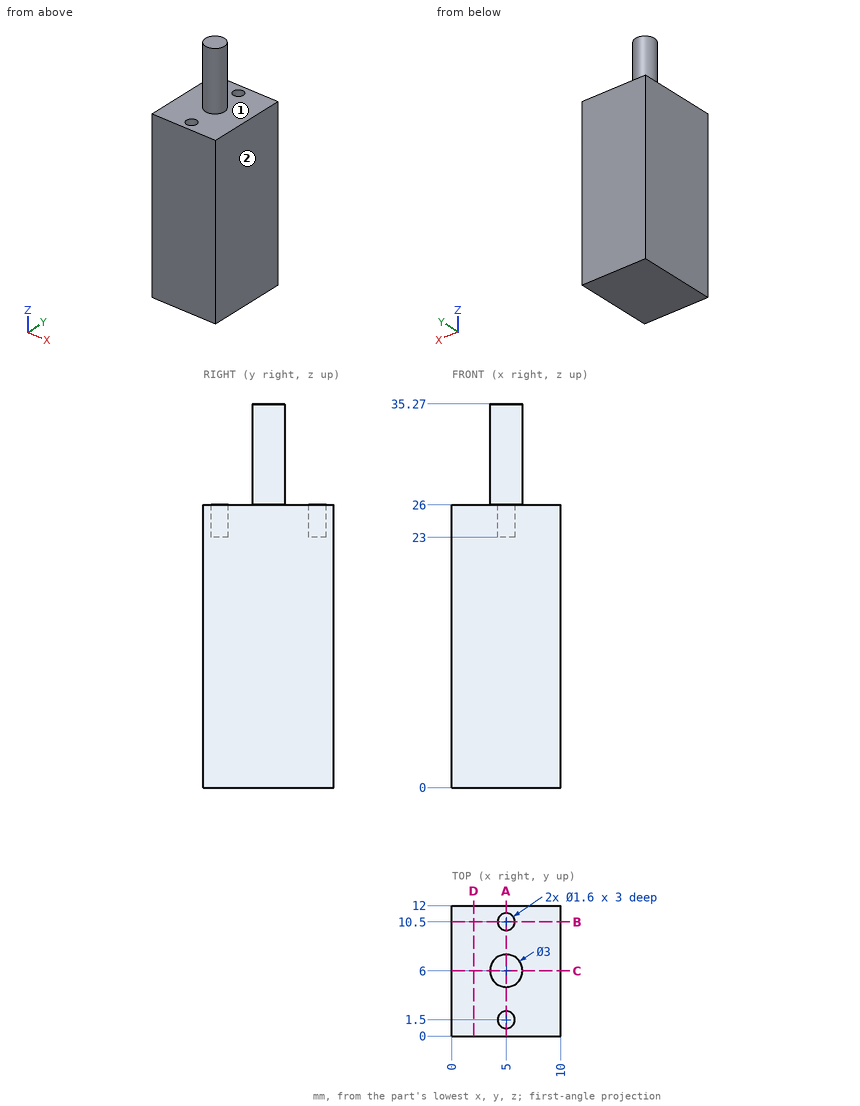
Here's the drawing with two shaded views (mm, measured from the low corner). I have some questions. A direction names the side the tool comes from. Coordinates: 2 decimals unless noted, no trailing zeros. Write each loop counter-clockwise with the first axis right and the second up, starting at its lowest first coordinate (ties: lowest second). Pieces come first, ordered by that corner, then holes. Notation, with made-up numbers: (4, -5) -> (49, -5) arc R34 ccw to (49, 34) -> close; hole circle Ø9 at (46.5, 20.5). An arc over 180 degrees is marked (long way). One line per question, with ' | ' between items. Start each with the question number.
1. If we section it at D-D (x = 2): Please give me the cut outline in (y, z).
2. Please list where these lines run through material, in increasing order: line 1 along Y through (x, z) = (5, 24.15); line 2 along Z through (x, y) = (6.25, 5); line 3 along X through (y, z) = (6.75, 26.5).
3. Will these pins go through, and if not, where does the flat tip stop? P1, Ø1.8, axis at x = 5, y = 10.5, coming from the +Z side; P2, Ø4, axis at y = 8, z = 31, coming from the -X side; P3, Ø3, axis at x = 3.5, y = 7.5, coming from the +Z side.
4. For the marked faces 1 and 2, which set-ups out of +Z, -Z, +X, -X, +Y, -Y let a thin tool reach every point of the face, with its end or its side?
5. If we section it at B-B (y = 10.5): Please give me the cut outline in (x, z), and give its area (3 significant figures).
6. If we section it at C-C (y = 6): Please give me the cut outline in (x, z).
7. If we section it at A-A (x = 5): Please give me the cut outline in (y, z).
Return value:
1) outline: (0, 0) -> (12, 0) -> (12, 26) -> (0, 26) -> close
2) line 1: y = 0 to 0.7, 2.3 to 9.7, 11.3 to 12 | line 2: z = 0 to 26 | line 3: x = 3.7 to 6.3
3) P1: stops at z = 26 | P2: stops at x = 3.5 | P3: stops at z = 35.27
4) face 1: +Z | face 2: +Z, -Z, +X, +Y, -Y
5) outline: (0, 0) -> (10, 0) -> (10, 26) -> (5.8, 26) -> (5.8, 23) -> (4.2, 23) -> (4.2, 26) -> (0, 26) -> close | area: 255 mm²
6) outline: (0, 0) -> (10, 0) -> (10, 26) -> (6.5, 26) -> (6.5, 35.27) -> (3.5, 35.27) -> (3.5, 26) -> (0, 26) -> close
7) outline: (0, 0) -> (12, 0) -> (12, 26) -> (11.3, 26) -> (11.3, 23) -> (9.7, 23) -> (9.7, 26) -> (7.5, 26) -> (7.5, 35.27) -> (4.5, 35.27) -> (4.5, 26) -> (2.3, 26) -> (2.3, 23) -> (0.7, 23) -> (0.7, 26) -> (0, 26) -> close
